Input: part model. Units: mm. Frame: model coordinates. Give positions to 0.01 mm unless a question says otherwise; leave off trailing zeros. Write each loop counter-clockwise with the first axis right and the second up, starting at its lowest first coordinate (ties: lowest second). Pieces come first, ordered by that corner, then holes. Notation, with made-up numbers: (4, -20.75) -> (27, -20.75) arc R31 ccw to (27, 5.25) -> close; hole circle Ø10 at (1.25, -26.75). An arc over 180 degrees is marked (long way). Return JSON: item names as keys, results as strings. Group by question number.
Item 1: Section D-D, the plane z = -12. Return loops of the section in (x, y), then the cut area to 3 significant figures.
Item 2: Section C-C, the plane y = 2.45. Count the separate pieces of the cut face and the enclosed holes in it, then the cut area to 3 significant figures.
Item 3: Section A-A, the plane z = 0. Return loops of the section in (x, y).
Item 4: Line query: line 1 (Z direction, x = 7.5, y = 4.2); line 2 (X direction, y = 2.35, z = 7.5); line 3 (Z direction, x = 7.5, y = 3.25). Output: solid intervals per line, ascending. Write a range as [from, to].
Item 5: Pin query (flat end, axial travel): P1, Ø1.4, axis at x = 7.5, z = -7.5, coming from the +Y side; P2, Ø3, axis at y = 2, z = -19, coming from the +X side; P3, Ø3, axis at x = 7.5, z = 7.5, coming from the +Y side. Return the tip coordinate at first contact, or that it passes through.
Item 6: Section B-B, the plane x = 0. Return loops of the section in (y, z).
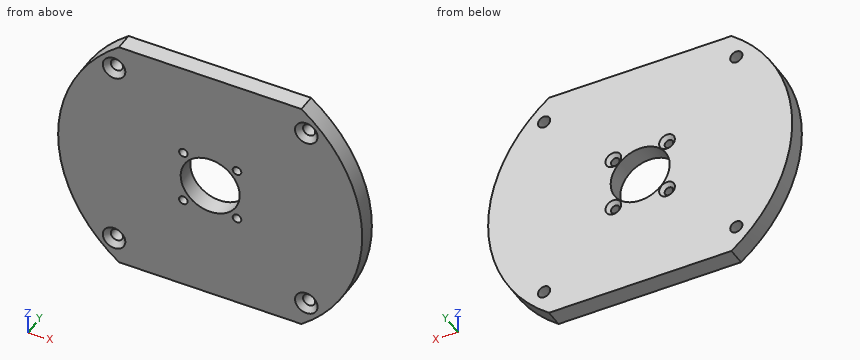
from build123d import *

# Parameters (mm, degrees)
SKETCH_1_R                   = 42.5
EXTRUDE_1_DEPTH              = 5
SKETCH_2_R                   = 8.25
CUT_EXTRUDE_1_DEPTH          = 61.311690409
HOLE_WIZARD_M2_1_D           = 2.4
HOLE_WIZARD_M2_1_CSINK_D     = 4.4
HOLE_WIZARD_M2_1_CSINK_ANGLE = 90
HOLE_WIZARD_M3_1_D           = 3.4
HOLE_WIZARD_M3_1_CSINK_D     = 6.3
HOLE_WIZARD_M3_1_CSINK_ANGLE = 90
PATTERN_CIRCULAR_1_COUNT     = 4
CUT_EXTRUDE_2_DEPTH          = 61.311690409


with BuildPart() as part:
    # Sketch 1 → Extrude 1 (new body)
    with BuildSketch(Plane(origin=(0, 0, 0), x_dir=(1, 0, 0), z_dir=(0, 1, 0))):
        with Locations(Location((0, 0, 0), (0, 0, 270))):
            Circle(SKETCH_1_R)
    extrude(amount=EXTRUDE_1_DEPTH)

    # Sketch 2 → Cut-Extrude 1 (cut, through all)
    with BuildSketch(Plane(origin=(0, 5, 0), x_dir=(1, 0, 0), z_dir=(0, 1, 0))):
        with Locations(Location((0, 0, 0), (0, 0, 270))):
            Circle(SKETCH_2_R)
    extrude(amount=-CUT_EXTRUDE_1_DEPTH, mode=Mode.SUBTRACT)

    # Hole Wizard M2 _1 (through all)
    with Locations(Plane(origin=(0, 5, 0), x_dir=(1, 0, 0), z_dir=(0, 1, 0))):
        with Locations((-7.5, 7.5), (7.5, 7.5), (7.5, -7.5), (-7.5, -7.5)):
            CounterSinkHole(HOLE_WIZARD_M2_1_D / 2, HOLE_WIZARD_M2_1_CSINK_D / 2, counter_sink_angle=HOLE_WIZARD_M2_1_CSINK_ANGLE)

    # Hole Wizard M3 _1 (through all)
    with Locations(Plane(origin=(0, 0, 0), x_dir=(-1, 0, 0), z_dir=(0, -1, 0))):
        with Locations((26.870057685, -26.870057685)):
            hole_wizard_m3_1 = CounterSinkHole(HOLE_WIZARD_M3_1_D / 2, HOLE_WIZARD_M3_1_CSINK_D / 2, counter_sink_angle=HOLE_WIZARD_M3_1_CSINK_ANGLE)

    # Pattern Circular 1: Hole Wizard M3 _1 ×4 about axis
    pattern_circular_1_axis = Axis((0, 0, 0), (0, 1, 0))
    for i in range(1, PATTERN_CIRCULAR_1_COUNT):
        add(hole_wizard_m3_1.rotate(pattern_circular_1_axis, i * 360 / PATTERN_CIRCULAR_1_COUNT), mode=Mode.SUBTRACT)

    # Sketch 7 → Cut-Extrude 2 (cut, symmetric)
    with BuildSketch(Plane(origin=(0, 5, 0), x_dir=(1, 0, 0), z_dir=(0, 1, 0))):
        Polygon((240.207107839, -34), (25.5, -34), (-25.5, -34), (-240.207107839, -34), (-240.207107839, -463.414215679), (240.207107839, -463.414215679), align=None)
    cut_extrude_2 = extrude(amount=CUT_EXTRUDE_2_DEPTH, both=True, mode=Mode.SUBTRACT)

    # Mirror 1: Cut-Extrude 2 across plane
    add(cut_extrude_2.mirror(Plane.XY), mode=Mode.SUBTRACT)


solid = part.part
Answer below:
{
 "1": {"outline": "(-40.77, 0) -> (40.77, 0) -> (40.77, 5) -> (-40.77, 5) -> close", "area": "408 mm2"},
 "2": {"separate pieces": "1", "enclosed holes": "9", "area": "4,820 mm2"},
 "3": {"outline": "(-42.5, 0) -> (-8.25, 0) -> (-8.25, 5) -> (-42.5, 5) -> close; (8.25, 0) -> (42.5, 0) -> (42.5, 5) -> (8.25, 5) -> close"},
 "4": {"line 1": "z = [-34, -8.9], [-6.1, -3.44], [3.44, 6.1], [8.9, 34]", "line 2": "x = [-41.83, -8.7], [-6.3, -3.44], [3.44, 6.3], [8.7, 41.83]", "line 3": "z = [-34, -8.7], [-6.3, -3.44], [3.44, 6.3], [8.7, 34]"},
 "5": {"P1": "passes through", "P2": "stops at x = 38.73", "P3": "stops at y = 4.3"},
 "6": {"outline": "(0, -34) -> (5, -34) -> (5, -8.25) -> (0, -8.25) -> close; (0, 8.25) -> (5, 8.25) -> (5, 34) -> (0, 34) -> close"}
}
